Read the model definition and answer for the solid it produces. Units are mm, in the model's axes. A direction names the side the tool comes from. Coordinates: 2 decimals unless noted, no trailing zeros. Write each loop counter-clockwise with the first axis right and the second up, starting at its lowest first coordinate (ties: lowest second). Pieces come first, ordered by that corner, then holes.
1) The part is cut by section D-D (x = 2.75). Determine the outline of the cut face in (y, z), then the cut area to 3 significant figures.
2) Determine the mould class of faces 1 (the face through (-2.44, 4.19, -0.54)), 2 (the face through (-2, 13.5, 6)), 3 (the face through (3.59, 12.51, 4.68)), 4 (the face through (-3.3, 16, 2.2)) for opening direction Z: +Z half, -Z half, draft (parallel to the pull), parting line (faces both ways), or undercut.
3) Find the intervals of material crossed by line 1 (Z direction, x = 0, y = 4.5); line 2 (X direction, y = 13, z = 0); line 3 (X direction, y = 16.25, z = 0), in increasing order.
4) The part is cut by section B-B (x = 0). Determine the outline of the cut face in (y, z).
5) The part is cut by section C-C (y = 8). Determine the outline of the cut face in (x, z), then the cut area to 3 significant figures.
6) Which of the six approach directions +Z, -Z, +X, -X, +Y, -Y give full straight-line access (tool end or side, diameter ignored) to faces 5 (the face through (-4.88, 16.51, -1.08)), 6 (the face through (-2, 11.5, 6)), 7 (the face through (2, 17, 5))?
7) The part is cut by section A-A (z = 0). Determine the outline of the cut face in (x, y), then the cut area to 3 significant figures.
8) Each of these flat-tipped pins is pushed along its axis until it touches: pin 1 Ø2 at (y, z) = (7, -3.5) entering from -X; pin 2 Ø1 at (x, y) = (-4.5, 4.5) entering from +Z; pin 3 Ø1.5 at (x, z) = (-1, 4) entering from +Y. Where does it stop, or does it pass through?
from build123d import *

# Parameters (mm, degrees)
SKETCH_1_R          = 6.9
SKETCH_1_R_2        = 2.5
EXTRUDE_1_DEPTH     = 17
SKETCH_2_R          = 3.5
CUT_EXTRUDE_1_DEPTH = 8.5
SKETCH_3_R          = 5
CUT_EXTRUDE_2_DEPTH = 1
SKETCH_4_W          = 2.072752753
SKETCH_4_H          = 2


with BuildPart() as part:
    # 草图1 → 凸台-拉伸1 (new body)
    with BuildSketch(Plane(origin=(0, 0, 0), x_dir=(1, 0, 0), z_dir=(0, 1, 0))):
        with Locations(Location((0, 0, 0), (0, 0, 270))):
            Circle(SKETCH_1_R)
        with Locations(Location((0, 0, 0), (0, 0, 270))):
            Circle(SKETCH_1_R_2, mode=Mode.SUBTRACT)
    extrude(amount=EXTRUDE_1_DEPTH)

    # 草图2 → 切除-拉伸1 (cut)
    with BuildSketch(Plane(origin=(0, 17, 0), x_dir=(1, 0, 0), z_dir=(0, 1, 0))):
        with Locations(Location((0, 0, 0), (0, 0, 270))):
            Circle(SKETCH_2_R)
    extrude(amount=-CUT_EXTRUDE_1_DEPTH, mode=Mode.SUBTRACT)

    # 草图3 → 切除-拉伸2 (cut)
    with BuildSketch(Plane(origin=(0, 17, 0), x_dir=(1, 0, 0), z_dir=(0, 1, 0))):
        with Locations(Location((0, 0, 0), (0, 0, 270))):
            Circle(SKETCH_3_R)
    extrude(amount=-CUT_EXTRUDE_2_DEPTH, mode=Mode.SUBTRACT)

    # 草图4 → 切除-旋转1 (revolve, cut)
    with BuildSketch(Plane.XY, mode=Mode.PRIVATE) as cut_revolve_1_sk:
        with Locations((6.936376377, 12.5)):
            Rectangle(SKETCH_4_W, SKETCH_4_H)
    revolve(cut_revolve_1_sk.sketch.rotate(Axis((0, 0, 0), (0, 1, 0)), 90), axis=Axis((0, 0, 0), (0, 1, 0)), mode=Mode.SUBTRACT)


solid = part.part
Reported:
1. outline: (0, -6.33) - (11.5, -6.33) - (11.5, -5.22) - (13.5, -5.22) - (13.5, -6.33) - (17, -6.33) - (17, -4.18) - (16, -4.18) - (16, -2.17) - (8.5, -2.17) - (8.5, 2.17) - (16, 2.17) - (16, 4.18) - (17, 4.18) - (17, 6.33) - (13.5, 6.33) - (13.5, 5.22) - (11.5, 5.22) - (11.5, 6.33) - (0, 6.33) - close
1. area: 170 mm2
2. face 1: undercut
2. face 2: draft
2. face 3: parting line
2. face 4: undercut
3. line 1: z = -6.9 to -2.5, 2.5 to 6.9
3. line 2: x = -5.9 to -3.5, 3.5 to 5.9
3. line 3: x = -6.9 to -5, 5 to 6.9
4. outline: (0, -6.9) - (11.5, -6.9) - (11.5, -5.9) - (13.5, -5.9) - (13.5, -6.9) - (17, -6.9) - (17, -5) - (16, -5) - (16, -3.5) - (8.5, -3.5) - (8.5, -2.5) - (0, -2.5) - close; (0, 2.5) - (8.5, 2.5) - (8.5, 3.5) - (16, 3.5) - (16, 5) - (17, 5) - (17, 6.9) - (13.5, 6.9) - (13.5, 5.9) - (11.5, 5.9) - (11.5, 6.9) - (0, 6.9) - close
5. outline: circle Ø13.8 at (0, 0); hole circle Ø5 at (0, 0)
5. area: 130 mm2
6. face 5: +Y
6. face 6: none
6. face 7: +Z, -Z, +X, -X, +Y
7. outline: (-6.9, 0) - (-2.5, 0) - (-2.5, 8.5) - (-3.5, 8.5) - (-3.5, 16) - (-5, 16) - (-5, 17) - (-6.9, 17) - (-6.9, 13.5) - (-5.9, 13.5) - (-5.9, 11.5) - (-6.9, 11.5) - close; (2.5, 0) - (6.9, 0) - (6.9, 11.5) - (5.9, 11.5) - (5.9, 13.5) - (6.9, 13.5) - (6.9, 17) - (5, 17) - (5, 16) - (3.5, 16) - (3.5, 8.5) - (2.5, 8.5) - close
7. area: 126 mm2
8. pin 1: stops at x = -6.43
8. pin 2: stops at z = 5.62
8. pin 3: stops at y = 16
